from build123d import *

# Parameters (mm, degrees)
SKIZZE2_W                      = 25
SKIZZE2_H                      = 25
SKIZZE2_R                      = 3.5
FRONT_FACE_DEPTH               = 1
SKIZZE3_W                      = 3.5
SKIZZE3_H                      = 26
SKIZZE3_R                      = 0.75
CAMERA_SPACER_DEPTH            = 4
FLOOR_PLATE_DEPTH              = 14
FLOOR_PLATE_DEPTH_BACK         = 0.5
SKIZZE6_W                      = 5
SKIZZE6_H                      = 2
SKIZZE7_W                      = 6
SKIZZE7_H                      = 26
SIDE_COVERS_DEPTH              = 0.5
TOP_COVER_REACH                = 34.669
SKIZZE8_W                      = 25
SKIZZE8_H                      = 1
FASE1_SIZE                     = 4.5
F_3_0_3_DURCHMESSER_BOHRUNG1_D = 3


with BuildPart() as part:
    # Skizze2 → Front Face (new body)
    # profile 1 of 2: a face of its own
    with BuildSketch(Plane(origin=(0, 0, 0), x_dir=(0, 0, -1), z_dir=(1, 0, 0))):
        with Locations((0, 12.5)):
            Rectangle(SKIZZE2_W, SKIZZE2_H)
        with Locations((0, 13)):
            Circle(SKIZZE2_R, mode=Mode.SUBTRACT)
    # profile 2 of 2: a face of its own
    with BuildSketch(Plane(origin=(0, 0, 0), x_dir=(0, 0, -1), z_dir=(1, 0, 0))):
        Polygon((12.5, 0), (-12.5, 0), (-17.5, 0), (-17.5, -1), (17.5, -1), (17.5, 0), align=None)
    extrude(amount=FRONT_FACE_DEPTH)

    # Skizze3 → Camera Spacer (add)
    # profile 1 of 2: a face of its own
    with BuildSketch(Plane.ZY):
        with Locations((-10.75, 12)):
            Rectangle(SKIZZE3_W, SKIZZE3_H)
        with Locations((-10.75, 14)):
            Circle(SKIZZE3_R, mode=Mode.SUBTRACT)
        with Locations((-10.75, 1.5)):
            Circle(SKIZZE3_R, mode=Mode.SUBTRACT)
    # profile 2 of 2: a face of its own
    with BuildSketch(Plane.ZY):
        with Locations((10.75, 12)):
            Rectangle(SKIZZE3_W, SKIZZE3_H)
        with Locations((10.75, 1.5)):
            Circle(SKIZZE3_R, mode=Mode.SUBTRACT)
        with Locations((10.75, 14)):
            Circle(SKIZZE3_R, mode=Mode.SUBTRACT)
    extrude(amount=CAMERA_SPACER_DEPTH)

    # Skizze6 → Floor Plate (add, two sides: drawn at the far end of the back side and taken through both)
    with BuildSketch(Plane.ZY.offset(-FLOOR_PLATE_DEPTH_BACK)):
        with Locations((-15, 0)):
            Rectangle(SKIZZE6_W, SKIZZE6_H)
        with Locations((15, 0)):
            Rectangle(SKIZZE6_W, SKIZZE6_H)
    extrude(amount=FLOOR_PLATE_DEPTH + FLOOR_PLATE_DEPTH_BACK)

    # Skizze7 → Side Covers (add)
    with BuildSketch(Plane(origin=(1, 0, 0), x_dir=(0, 0, -1), z_dir=(1, 0, 0))):
        with Locations((15.5, 12)):
            Rectangle(SKIZZE7_W, SKIZZE7_H)
        with Locations((-15.5, 12)):
            Rectangle(SKIZZE7_W, SKIZZE7_H)
    extrude(amount=-SIDE_COVERS_DEPTH)

    # Top Cover: up to this face of the body (flat: up to its plane)
    top_cover_end = Plane(part.part.faces().sort_by_distance((0.5, 12.821917808, -15.534246575))[0])
    # Skizze8 → Top Cover (cut, up to the picked face)
    with BuildSketch(Plane.ZY.offset(4), mode=Mode.PRIVATE) as top_cover_sk1:
        with Locations((0, 24.5)):
            Rectangle(SKIZZE8_W, SKIZZE8_H)
    top_cover_tool1 = split(extrude(top_cover_sk1.sketch, amount=-TOP_COVER_REACH, mode=Mode.PRIVATE), bisect_by=top_cover_end, keep=Keep.BOTH, mode=Mode.PRIVATE)
    add(top_cover_tool1.solids().sort_by(Axis((-4, 24.5, 0), (1, 0, 0)))[0], mode=Mode.SUBTRACT)

    # Fase1
    fase1_edges = [part.edges().sort_by_distance(p)[0] for p in [
        (0.5, 1, 15),
        (0.5, 1, -15),
    ]]
    chamfer(fase1_edges, length=FASE1_SIZE)

    # Ø3.0 (3) Durchmesser Bohrung1 (through all)
    with Locations(Plane(origin=(0, 1, 0), x_dir=(1, 0, 0), z_dir=(0, 1, 0))):
        with Locations((-11, 15), (-11, -15)):
            Hole(F_3_0_3_DURCHMESSER_BOHRUNG1_D / 2)


solid = part.part
Work out the finished part from the listing and answer in its coordinate system (mm). A direction names the side the tool comes from. Round coordinates to 2 decimals unless told otherwise and drop trailing zeros. Write each loop counter-clockwise with the first axis right and the second up, starting at its lowest first coordinate (ties: lowest second). Pieces come first, ordered by that corner, then holes. Notation, with made-up numbers: M -15,26 L 7,26 A21 ccw 7,33 Z; hole C -3.5,-5.75 d5. An arc over 180 degrees is marked long. Use a Markdown table: item, result.
1) The part is cut by section B-B on z = 15. Give the vertices of the cut face in (x, y).
Taken from the geometry:
| item | result |
|---|---|
| outline | M -14,-1 L -12.5,-1 L -12.5,1 L -14,1 Z; M -9.5,-1 L 1,-1 L 1,25 L 0.5,25 L 0.5,5.5 L -4,1 L -9.5,1 Z |
2) The part is cut by section D-D on x = -11. Give the vertices of the cut face in (y, z).
Taken from the geometry:
| item | result |
|---|---|
| outline | M -1,-17.5 L 1,-17.5 L 1,-16.5 L -1,-16.5 Z; M -1,-13.5 L 1,-13.5 L 1,-12.5 L -1,-12.5 Z; M -1,12.5 L 1,12.5 L 1,13.5 L -1,13.5 Z; M -1,16.5 L 1,16.5 L 1,17.5 L -1,17.5 Z |
3) The part is cut by section A-A on x = -2.25. Give the vertices of the cut face in (y, z).
Taken from the geometry:
| item | result |
|---|---|
| outline | M -1,-17.5 L 2.75,-17.5 L 2.75,-12.5 L 24,-12.5 L 24,-9 L -1,-9 Z; M -1,9 L 24,9 L 24,12.5 L 2.75,12.5 L 2.75,17.5 L -1,17.5 Z; hole C 1.5,-10.75 d1.5; hole C 1.5,10.75 d1.5; hole C 14,-10.75 d1.5; hole C 14,10.75 d1.5 |
4) Which of the six approach directions +Z, -Z, +X, -X, +Y, -Y give full straight-line access (tool end or side, diameter ignored) to faces 4 (the face through (-2, 11, 9)), 5 (the face through (-2, 3, 15)), 6 (the face through (-9, 1, -15)), 7 (the face through (0, 14, 11))?
Taken from the geometry:
| item | result |
|---|---|
| face 4 | -X, +Y, -Y |
| face 5 | +Z, -X, +Y |
| face 6 | +Z, -Z, -X, +Y |
| face 7 | -X |
5) Flat-ended cylindrical pins translate along their axes: pin 1 (0.8 mm diameter, centred on y = 13.5, z = 10.5, fed in from -X); pin 2 (5 mm diameter, centred on x = -6, y = 4, fed in from -Z); pin 3 (4.5 mm diameter, centred on x = -3, y = 14.5, fed in from +Z). Find the tip coordinate at first contact, or state that the pin passes through.
Taken from the geometry:
| item | result |
|---|---|
| pin 1 | stops at x = -4 |
| pin 2 | stops at z = -12.5 |
| pin 3 | stops at z = 12.5 |
6) Determine the mould class of faces 1 (the face through (-5.24, 0.85, 17.5)), 2 (the face through (0.3, -1, -4.4)), 3 (the face through (-1.972, 14.744, 10.652)) for opening direction Z: pulls with the +Z half, pulls with the -Z half, needs draft (parallel to the pull), parting line crosses it, or undercut.
Taken from the geometry:
| item | result |
|---|---|
| face 1 | pulls with the +Z half |
| face 2 | needs draft |
| face 3 | undercut |
7) The part is cut by section C-C on y = 1.5. Give the vertices of the cut face in (x, z).
Taken from the geometry:
| item | result |
|---|---|
| outline | M -4,-12.5 L -3.5,-12.5 L -3.5,-17.5 L 0.5,-17.5 L 0.5,-18.5 L 1,-18.5 L 1,18.5 L 0.5,18.5 L 0.5,17.5 L -3.5,17.5 L -3.5,12.5 L -4,12.5 L -4,11.5 L 0,11.5 L 0,10 L -4,10 L -4,9 L 0,9 L 0,-9 L -4,-9 L -4,-10 L 0,-10 L 0,-11.5 L -4,-11.5 Z |
8) Consider line 1 (Z direction, x = -11, y = -0.05); line 2 (Y direction, x = -0.8, z = 10.75); line 3 (Z direction, x = -1, y = 17.25). Determine where each line is inside the solid, lowest interval first. Write a range as [from, to].
Taken from the geometry:
| item | result |
|---|---|
| line 1 | z = [-17.5, -16.5], [-13.5, -12.5], [12.5, 13.5], [16.5, 17.5] |
| line 2 | y = [-1, 0.75], [2.25, 13.25], [14.75, 24] |
| line 3 | z = [-12.5, -9], [9, 12.5] |
